Source: CAD feature listing. Evaluate the final solid. Frame: model axes, mm. Give positions to 0.01 mm unless a question says otherwise; leave off trailing zeros. Write each loop counter-clockwise with the first axis right and the second up, starting at its lowest first coordinate (ties: lowest second). Pieces come first, ordered by that corner, then holes. Notation, with made-up numbers: (-10, 29.25) -> (-4, 29.25) arc R27 ccw to (-4, 52.25) -> close; hole circle Ø2 at (-35, 24). An arc over 180 degrees is marked (long way). Use one line per item in the form item = value. Start each with the question number.
(1) Cut plane A-A, the plane z = -73. Output: boundary loops of the cut face in (x, y), and give its area (3 significant figures).
(2) Cut plane C-C, the plane x = -40. Output: boundary loops of the cut face in (y, z).
(3) Cut plane B-B, the plane y = 0.75. Output: boundary loops of the cut face in (x, z) (3 decimals), and give its area (3 significant figures).
(4) Material intervals for line 1 along Z through (x, y) = (-40, 0.2), sorted ascending. Write a range as from..to.
Autodesk Inventor part; units mm, degrees
ref_plane "YZ Plane" through (0, 0, 0) normal (1, 0, 0) x (0, 1, 0)
ref_plane "XZ Plane" through (0, 0, 0) normal (0, 1, 0) x (-1, 0, 0)
ref_plane "XY Plane" through (0, 0, 0) normal (0, 0, 1) x (1, 0, 0)
sketch "Sketch1" plane through (0, 0, 0) normal (0, 1, 0) x (-1, 0, 0)
  line L0 (0, 0) -> (45, 0)
  line L1 (45, 0) -> (45, -83)
  line L2 (45, -83) -> (0, -83)
  line L3 (0, -83) -> (0, 0)
  circle A0 centre (39, -73) radius 2
  line L4 (22.5, 0) -> (22.5, -83)
  circle A1 centre (6, -73) radius 2
  line L5 (45, -10) -> (0, -10)
  line L6 (6, -3.5) -> (11.525, -3.5)
  line L7 (11.525, -3.5) -> (11.525, -5)
  line L8 (11.525, -5) -> (6, -5)
  line L9 (6, -5) -> (6, -3.5)
  line L10 (6, -16.5) -> (11.525, -16.5)
  line L11 (11.525, -16.5) -> (11.525, -15)
  line L12 (11.525, -15) -> (6, -15)
  line L13 (6, -15) -> (6, -16.5)
  line L14 (39, -3.5) -> (33.475, -3.5)
  line L15 (33.475, -3.5) -> (33.475, -5)
  line L16 (33.475, -5) -> (39, -5)
  line L17 (39, -5) -> (39, -3.5)
  line L18 (39, -16.5) -> (33.475, -16.5)
  line L19 (33.475, -15) -> (39, -15)
  line L20 (39, -15) -> (39, -16.5)
  line L21 (33.475, -16.5) -> (33.475, -15)
  dimension "d0" = 45
  dimension "d1" = 83
  dimension "d2" = 10
  dimension "d3" = 6
  dimension "d9" = 4
  dimension "d13" = 45
  dimension "d22" = 20
  dimension "d23" = 6
  dimension "d24" = 10
  dimension "d25" = 1.5
extrude "Extrusion3" add sketch "Sketch1" along normal blind 1
equation "\"d13\" = d0"
properties part number "Platte1"
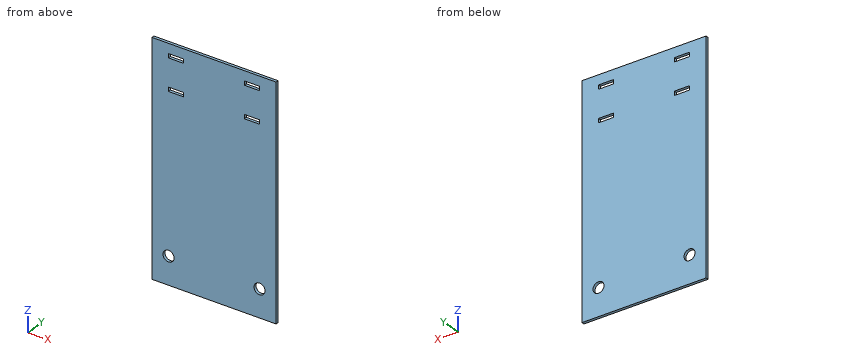
Geometry says:
q1.outline = (-45, 0) -> (-41, 0) -> (-41, 1) -> (-45, 1) -> close; (-37, 0) -> (-8, 0) -> (-8, 1) -> (-37, 1) -> close; (-4, 0) -> (0, 0) -> (0, 1) -> (-4, 1) -> close
q1.area = 37.0 mm^2
q2.outline = (0, -83) -> (1, -83) -> (1, -74.73) -> (0, -74.73) -> close; (0, -71.27) -> (1, -71.27) -> (1, 0) -> (0, 0) -> close
q3.outline = (-45, -83) -> (0, -83) -> (0, 0) -> (-45, 0) -> close; hole circle Ø4 at (-39, -73); hole (-39, -16.5) -> (-33.475, -16.5) -> (-33.475, -15) -> (-39, -15) -> close; hole (-39, -5) -> (-33.475, -5) -> (-33.475, -3.5) -> (-39, -3.5) -> close; hole (-11.525, -16.5) -> (-6, -16.5) -> (-6, -15) -> (-11.525, -15) -> close; hole (-11.525, -5) -> (-6, -5) -> (-6, -3.5) -> (-11.525, -3.5) -> close; hole circle Ø4 at (-6, -73)
q3.area = 3,680 mm^2
q4.line_1 = -83..-74.73, -71.27..0
